from build123d import *

# Parameters (mm, degrees)
SKETCH1_W           = 500
SKETCH1_H           = 500
SKETCH1_R           = 55
SKETCH1_R_2         = 5
BOSS_EXTRUDE1_DEPTH = 10


with BuildPart() as part:
    # Sketch1 → Boss-Extrude1 (new, symmetric)
    with BuildSketch(Plane(origin=(0, 0, 0), x_dir=(1, 0, 0), z_dir=(0, 1, 0))):
        Rectangle(SKETCH1_W, SKETCH1_H)
        with Locations(Location((0, 0, 0), (0, 0, 270))):
            Circle(SKETCH1_R, mode=Mode.SUBTRACT)
        with Locations(Location((-150, 150, 0), (0, 0, 270))):
            Circle(SKETCH1_R_2, mode=Mode.SUBTRACT)
        with Locations(Location((150, 150, 0), (0, 0, 270))):
            Circle(SKETCH1_R_2, mode=Mode.SUBTRACT)
        with Locations(Location((-150, -150, 0), (0, 0, 270))):
            Circle(SKETCH1_R_2, mode=Mode.SUBTRACT)
        with Locations(Location((150, -150, 0), (0, 0, 270))):
            Circle(SKETCH1_R_2, mode=Mode.SUBTRACT)
    extrude(amount=BOSS_EXTRUDE1_DEPTH, both=True)


solid = part.part
Input: part model. Units: mm. Frame: model coordinates. Give positions to 0.01 mm unless a question says otherwise; leave off trailing zeros. Write each loop counter-clockwise with the first axis right and the second up, starting at its lowest first coordinate (ties: lowest second). Pieces come first, ordered by that corner, then holes. Notation, with made-up numbers: M -34,9 L -24,9 A20 cw -24,37 Z; hole C -28.5,-0.5 d6. An arc over 180 degrees is marked long. Write item = value, one per line. Start each with the question number.
1) Cut plane B-B on x = 0. Return the cut outline in (y, z), then the cut area to 3 significant figures.
2) Cut plane A-A on z = 0. Return the cut outline in (x, y), then the cut area to 3 significant figures.
3) Cut plane C-C on y = 2. Return the cut outline in (x, z).
4) Material intervals for line 1 along X through (y, z) = (-0.75, 150); line 2 along X through (y, z) = (-1.25, 0); line 3 along X through (y, z) = (-8, -43), sorted ascending. Write a range as [from, to].
5) Draft query along X for faces 1 (the cylindrical face through (-48.794, -0.14, 25.379)), 2 (the flat face through (-250, 0, 3)), 3 (the flat face through (-3, 0, -250)). Return one class per face: +X half, -X half, draft (parallel to the pull), parting line (faces both ways), or undercut.
Solved:
q1.outline = M -10,-250 L 10,-250 L 10,-55 L -10,-55 Z; M -10,55 L 10,55 L 10,250 L -10,250 Z
q1.area = 7,800 mm2
q2.outline = M -250,-10 L -55,-10 L -55,10 L -250,10 Z; M 55,-10 L 250,-10 L 250,10 L 55,10 Z
q2.area = 7,800 mm2
q3.outline = M -250,-250 L 250,-250 L 250,250 L -250,250 Z; hole C -150,-150 d10; hole C -150,150 d10; hole C 0,0 d110; hole C 150,-150 d10; hole C 150,150 d10
q4.line_1 = [-250, -155], [-145, 145], [155, 250]
q4.line_2 = [-250, -55], [55, 250]
q4.line_3 = [-250, -34.29], [34.29, 250]
q5.face_1 = undercut
q5.face_2 = -X half
q5.face_3 = draft
